```python
from build123d import *

# Parameters (mm, degrees)
F0_W     = 56.4
F0_H     = 56.4
F0_R     = 2.914102
F0_R_2   = 22.195946
F1_DEPTH = 5
F2_W     = 56.4
F2_H     = 49
F2_R     = 3
F3_DEPTH = 5
F4_R     = 3


with BuildPart() as f1:
    # F0 (on Top) → F1 (new body)
    with BuildSketch(Plane.XY):
        Rectangle(F0_W, F0_H)
        with Locations((-23.57, -23.57)):
            Circle(F0_R, mode=Mode.SUBTRACT)
        with Locations((23.57, -23.57)):
            Circle(F0_R, mode=Mode.SUBTRACT)
        Circle(F0_R_2, mode=Mode.SUBTRACT)
        with Locations((-23.57, 23.57)):
            Circle(F0_R, mode=Mode.SUBTRACT)
        with Locations((23.57, 23.57)):
            Circle(F0_R, mode=Mode.SUBTRACT)
        Polygon((28.203152, -28.2), (28.2, -28.2), (-28.2, -28.2), (-28.2, -33.2), (28.203152, -33.2), align=None)
    extrude(amount=F1_DEPTH)

    # F2 (on face) → F3 (join)
    with BuildSketch(Plane.XZ.offset(33.2)):
        with Locations((0, -24.5)):
            Rectangle(F2_W, F2_H)
        with Locations((-23.57, -43.577386)):
            Circle(F2_R, mode=Mode.SUBTRACT)
        with Locations((23.57, -43.577386)):
            Circle(F2_R, mode=Mode.SUBTRACT)
        with Locations((-23.57, -6.577386)):
            Circle(F2_R, mode=Mode.SUBTRACT)
        with Locations((23.57, -6.577386)):
            Circle(F2_R, mode=Mode.SUBTRACT)
    extrude(amount=-F3_DEPTH)

    # F4
    f4_edges = [f1.edges().sort_by_distance(p)[0] for p in [
        (-28.2, 28.2, 2.5),
        (28.2, 28.2, 2.5),
        (-28.2, -30.7, -49),
        (28.2, -30.7, -49),
    ]]
    fillet(f4_edges, radius=F4_R)


solid = f1.part
```
Part model, mm, in its own coordinate system. A direction names the side the tool comes from. Give positions to 0.01 mm unless a question says otherwise; leave off trailing zeros. Order: outer loops, then holes, each group sorted by start corner. A loop starts at its lowest first (then second) coordinate and runs counter-clockwise, first axis right, second up. Notation, with made-up numbers: M 75,72 L 80,72 A37 cw 80,110 Z; hole C 66,65.25 d1. An arc over 180 degrees is marked long. Use a Markdown table: item, result. Add a question column.
(1) Saw through at A-A, the plane x = 0. Give the cut face in (y, z).
(2) Mould opens along Z. For faces 3 (the face through (21.189, -30.735, -8.403)), 4 (the face through (28.203, -31, 2)), 5 (the face through (0, -23, 5)), 6 (the face through (-13, 19, 0)) say: +Z half, -Z half, draft (parallel to the pull), parting line (faces both ways), or undercut.
(3) Saw through at C-C, the plane x = -23.57. Give the cut face in (y, z).
(4) Saw through at B-B, the plane y = 0. Give the cut face in (x, z).
(5) Saw through at D-D, the plane y = 23.57. Give the cut face in (x, z), and give its area (3 significant figures).
(6) Probe line 1 along Z through (x, y) = (-23.57, -30.25); line 2 along Y through (x, z) = (23.57, 1.95); line 3 along Y through (x, z) = (0, 2). List the from-to ranges inside material, lowest first. Write a range as [from, to].
(7) 3-axis set-ups, long thin cutter, end or side, ignore diameter. For faces 1 (the face through (0, -28.2, -24)), 2 (the face through (28.2, -2, 2)): which of +Z, -Z, +X, -X, +Y, -Y reach the whole face in a straight line?
(8) Drop flat-ended pins along their axis: P1, Ø4, axis at y = -31, z = -28, coming from the +X side; P2, Ø5, axis at x = 23.57, z = -6.58, coming from the -Y side; P3, Ø8, axis at x = -4, z = -15.5, coming from the +Y side; P4, Ø7.5, axis at x = -23.57, y = 23.57, coming from the -Z side. Give the stop position or say it passes through.
Answer key:
| question | item | result |
|---|---|---|
| 1 | outline | M -33.2,-49 L -28.2,-49 L -28.2,0 L -22.2,0 L -22.2,5 L -33.2,5 Z; M 22.2,0 L 28.2,0 L 28.2,5 L 22.2,5 Z |
| 2 | face 3 | undercut |
| 2 | face 4 | draft |
| 2 | face 5 | +Z half |
| 2 | face 6 | -Z half |
| 3 | outline | M -33.2,-49 L -28.2,-49 L -28.2,-46.58 L -33.2,-46.58 Z; M -33.2,-40.58 L -28.2,-40.58 L -28.2,-9.58 L -33.2,-9.58 Z; M -33.2,-3.58 L -28.2,-3.58 L -28.2,0 L -26.48,0 L -26.48,5 L -33.2,5 Z; M -20.66,0 L 20.66,0 L 20.66,5 L -20.66,5 Z; M 26.48,0 L 28.2,0 L 28.2,5 L 26.48,5 Z |
| 4 | outline | M -28.2,0 L -22.2,0 L -22.2,5 L -28.2,5 Z; M 22.2,0 L 28.2,0 L 28.2,5 L 22.2,5 Z |
| 5 | outline | M -28.2,0 L -26.48,0 L -26.48,5 L -28.2,5 Z; M -20.66,0 L 20.66,0 L 20.66,5 L -20.66,5 Z; M 26.48,0 L 28.2,0 L 28.2,5 L 26.48,5 Z |
| 5 | area | 224 mm^2 |
| 6 | line 1 | [-49, -46.58], [-40.58, -9.58], [-3.58, 5] |
| 6 | line 2 | [-33.2, -26.48], [-20.66, 20.66], [26.48, 28.2] |
| 6 | line 3 | [-33.2, -22.2], [22.2, 28.2] |
| 7 | face 1 | -Z, +X, -X, +Y |
| 7 | face 2 | +Z, -Z, +X, +Y, -Y |
| 8 | P1 | x = 28.2 |
| 8 | P2 | through |
| 8 | P3 | y = -28.2 |
| 8 | P4 | z = 0 |
